```python
from build123d import *

# Parameters (mm, degrees)
SKETCH2_W = 10
SKETCH2_H = 2


with BuildPart() as part:
    # Sweep1: sweep along a path in Sketch1
    with BuildLine(Plane(origin=(0, 0, 0), x_dir=(0, 0, -1), z_dir=(1, 0, 0))) as sweep1_path:
        Line((-45.581395349, 0), (-35, 0))
        ThreePointArc((-35, 0), (-31.464466094, 1.464466094), (-30, 5))
        Line((-30, 5), (-30, 20))
        ThreePointArc((-30, 20), (-28.535533906, 23.535533906), (-25, 25))
        Line((-25, 25), (25, 25))
        ThreePointArc((25, 25), (28.535533906, 23.535533906), (30, 20))
        Line((30, 20), (30, 5))
        ThreePointArc((30, 5), (31.464466094, 1.464466094), (35, 0))
        Line((35, 0), (45.581395349, 0))
    # Sketch2 → Sweep1 (sweep)
    with BuildSketch(Plane.XY.offset(45.581395349)):
        Rectangle(SKETCH2_W, SKETCH2_H)
    sweep(path=sweep1_path.line)

    # Sketch3 → Revolve1 (revolve)
    with BuildSketch(Plane(origin=(0, 0, 0), x_dir=(0, 0, -1), z_dir=(1, 0, 0)), mode=Mode.PRIVATE) as revolve1_sk:
        with BuildLine():
            Line((-25, 25), (-25, 26))
            ThreePointArc((-25, 26), (-23.535533906, 29.535533906), (-20, 31))
            Line((-20, 31), (20, 31))
            ThreePointArc((20, 31), (23.535533906, 29.535533906), (25, 26))
            Line((25, 26), (25, 25))
            Line((25, 25), (-25, 25))
        make_face()
    revolve(revolve1_sk.sketch.rotate(Axis((0, 25, -25), (0, 0, 1)), 90), axis=Axis((0, 25, -25), (0, 0, 1)))


solid = part.part
```
Geometry: final body of the model. Coordinates: model frame, mm. A direction names the side the tool comes from. Round coordinates to 2 decimals unless told otherwise and drop trailing zeros. Order: outer loops, then holes, each group sorted by start corner. A loop starts at its lowest first (then second) coordinate and runs counter-clockwise, first axis right, second up. Notation, with made-up numbers: (13, 51.5) - (36, 51.5) arc R17 ccw to (36, 81.5) - close; hole circle Ø7 at (35.25, 43.25). An arc over 180 degrees is marked (long way). Use CSV: the item, a comma, the result in double quotes. Start each with the question number.
Q1. Material intervals for line 1 along Z through (x, y) = (1, 16); line 2 along Y through (x, z) = (3.25, -40); line 3 along Z through (x, y) = (0.25, 21), sorted ascending. Write a range as from..to.
Q2. Access query for faces 1 (the face through (5, 9, -30)), 2 (the face through (4, 26, 24.4)), 3 (the face through (4, 24, -24.4)). Directions: +Z, -Z, +X, -X, +Y, -Y. A direction counts if a zero-diameter tool reaches every point of the face in a straight line with its end or side. Return the directions, or none.
Q3. First-contact query: pin 1 (5 mm diameter, centred on y = 21, z = -4, fed in from +X); pin 2 (18 mm diameter, centred on y = 18.5, z = -31, fed in from -X); pin 3 (5 mm diameter, centred on x = -2, y = 5.5, fed in from +Z). Flat tips, straight axial feed; report the tip coordinate or a pass-through.
Q4. Section query A-A (y = 12.5). Return loops of the section in (x, z), and give its area (3 significant figures).
Q5. Mould query, pull axis Z, two halves, no side actions, for faces 4 (the face through (0.07, 0.804, -30.711)), 5 (the face through (0, -1, -40)), 6 (the face through (0, 0, -45.581)), 7 (the face through (0, 13, 29)). Classes: +Z half, -Z half, draft (parallel to the pull), parting line (faces both ways), or undercut.
Q6. Section query B-B (z = 5). Return loops of the section in (x, y).
Q7. Section query C-C (y = 3). Return loops of the section in (x, z).
Result set:
1,line 1,"z = -31..-29, 29..31"
1,line 2,"y = -1..1"
1,line 3,"z = -30.92..-28.87, -23.99..23.99, 28.87..30.92"
2,face 1,"-Z, +X, +Y, -Y"
2,face 2,"+Z, +X, +Y"
2,face 3,"+X, -Y"
3,pin 1,"stops at x = 5.81"
3,pin 2,"stops at x = -5"
3,pin 3,"stops at z = 31.54"
4,outline,"(-5, -31) - (5, -31) - (5, -29) - (-5, -29) - close; (-5, 29) - (5, 29) - (5, 31) - (-5, 31) - close"
4,area,"40.0 mm2"
5,face 4,"undercut"
5,face 5,"draft"
5,face 6,"-Z half"
5,face 7,"undercut"
6,outline,"circle Ø12 at (0, 25)"
7,outline,"(-5, -31.54) - (5, -31.54) - (5, -29.34) - (-5, -29.34) - close; (-5, 29.34) - (5, 29.34) - (5, 31.54) - (-5, 31.54) - close"
